For this review, take the finished solid that the model builds, in its own axes (mm). A direction names the side the tool comes from. Give positions to 0.01 mm unless a question says otherwise; leave off trailing zeros. Write each loop counter-clockwise with the first axis right and the second up, starting at its lowest first coordinate (ties: lowest second). Pieces come first, ordered by that corner, then holes. Notation, with made-up numbers: M -35.5,-2 L 23.5,-2 A14 cw 23.5,7 Z; hole C 5,41 d6. An arc over 180 degrees is marked long. Write item = value, one per line.
Autodesk Inventor part; units mm, degrees
ref_plane "YZ Plane" through (0, 0, 0) normal (1, 0, 0) x (0, 1, 0)
ref_plane "XZ Plane" through (0, 0, 0) normal (0, 1, 0) x (-1, 0, 0)
ref_plane "XY Plane" through (0, 0, 0) normal (0, 0, 1) x (1, 0, 0)
sketch "Boceto1" plane through (0, 0, 0) normal (0, 0, 1) x (1, 0, 0)
  line L0 (-32, -32) -> (32, -32)
  line L1 (32, -32) -> (32, 32)
  line L2 (32, 32) -> (-32, 32)
  line L3 (-32, 32) -> (-32, -32)
  line L4 (-32, -32) -> (32, 32) construction
  line L5 (32, -32) -> (-32, 32) construction
  point P0 (0, 0)
  dimension "d0" = 64
  dimension "d1" = 64
extrude "Extrusión1" add sketch "Boceto1" along normal blind 3
sketch "Boceto2" plane through (32, -32, 0) normal (1, 0, 0) x (0, 0, -1)
  line L0 (-74, 16.5) -> (1, 16.5)
  arc A0 (1, 10.5) -> (1, 16.5) centre (1, 13.5) ccw
  line L1 (1, 10.5) -> (-74, 10.5)
  line L2 (-74, -4.5) -> (-74, 10.5)
  line L3 (7, -4.5) -> (-74, -4.5)
  line L4 (7, -4.5) -> (7, 68.5)
  line L5 (7, 68.5) -> (-74, 68.5)
  line L6 (-74, 53.5) -> (-74, 68.5)
  line L7 (-74, 53.5) -> (1, 53.5)
  arc A1 (1, 47.5) -> (1, 53.5) centre (1, 50.5) ccw
  line L8 (1, 47.5) -> (-74, 47.5)
  line L9 (-74, 16.5) -> (-74, 47.5)
  line L10 (0, 0) -> (0, 64)
  line L11 (0, 64) -> (-3, 64)
  line L12 (-3, 0) -> (-3, 64)
  line L13 (0, 0) -> (-3, 0)
  line L14 (0, 47.5) -> (-3, 47.5)
  line L15 (-3, 47.5) -> (-3, 53.5)
  line L16 (-3, 53.5) -> (0, 53.5)
  line L17 (0, 53.5) -> (0, 47.5)
  line L18 (0, 47.7) -> (-3, 47.7)
  line L19 (-2.8, 47.7) -> (-2.8, 53.3)
  line L20 (-3, 53.3) -> (0, 53.3)
  line L21 (-0.2, 53.3) -> (-0.2, 47.7)
  line L22 (-2.5, 53) -> (-2.5, 48)
  line L23 (-3, 48) -> (0, 48)
  line L24 (-0.5, 48) -> (-0.5, 53)
  line L25 (0, 53) -> (-3, 53)
  point P0 (0, 32)
  dimension "d4" = 0.2
  dimension "d10" = 0.5
extrude "Extrusión2" add sketch "Boceto2" along normal blind 10 contours L12 L25 L19 L23 | L23 L21 L25 L10 | L19 L25 L22 L23 | L23 L24 L25 L21 | L22 L25 L24 L23
sketch "Boceto3" plane through (42, -32, 0) normal (1, 0, 0) x (0, 0, -1)
  line L0 (-3, 53) -> (-3, 48)
  line L1 (0, 48) -> (0, 53)
  line L2 (0, 47.7) -> (-3, 53.3)
  circle A0 centre (-1.5, 50.5) radius 5
  line L3 (-3, 53.3) -> (-3, 55.2697)
  line L4 (-3, 47.7) -> (0, 47.7)
  line L5 (0, 47.7) -> (0, 53.3)
  line L6 (0, 53.3) -> (-3, 53.3)
  line L7 (-3, 53.3) -> (-3, 47.7)
  line L8 (-3, 47.7) -> (-3, 42)
  line L9 (-3, 48) -> (0, 48)
  line L10 (0, 53) -> (-3, 53)
  point P0 (0, 32)
  point P1 (-3, 45.7303)
  point P2 (-2.8393, 53)
  point P3 (-0.1607, 48)
  dimension "d7" = 10
extrude "Extrusión3" add sketch "Boceto3" along normal blind 3 contours L10 L2 L9 L0 | L7 L2 L10 | L9 L2 L4 L7 | L6 L5 L10 L2 | L3 A0 L8 L4 L5 L1 L6 | L10 L1 L9 L2 | L9 L5 L2
ref_plane "Plano de trabajo1" through (0, -32, 3) normal (1, 0, 0) x (0, 0, -1)
ref_plane "Plano de trabajo2" through (-32, 0, 0) normal (0, 1, 0) x (1, 0, 0)
mirror "Simetría1" about plane through (-32, 0, 0) normal (0, 1, 0) of "Extrusión2", "Extrusión3"
mirror "Simetría2" about plane through (0, -32, 3) normal (1, 0, 0) of "Extrusión2", "Simetría1", "Extrusión3"
sketch "Boceto4" plane through (0, 0, 3) normal (0, 0, 1) x (1, 0, 0)
  arc A0 (-26.7524, -33.5) -> (-33.5, -26.7524) centre (-31.4, -31.4) ccw
  arc A1 (33.5, -26.7524) -> (26.7524, -33.5) centre (31.4, -31.4) ccw
  arc A2 (26.7524, 33.5) -> (33.5, 26.7524) centre (31.4, 31.4) ccw
  arc A3 (-33.5, 26.7524) -> (-26.7524, 33.5) centre (-31.4, 31.4) ccw
  line L0 (32, -32) -> (32, -21)
  line L1 (32, -21) -> (42, -21)
  line L2 (42, -23.2697) -> (42, -21)
  line L3 (42, -23.2697) -> (45, -23.2697)
  line L4 (45, -23.2697) -> (45, -13.7303)
  line L5 (42, -13.7303) -> (45, -13.7303)
  line L6 (42, -16) -> (42, -13.7303)
  line L7 (32, -16) -> (42, -16)
  line L8 (32, -16) -> (32, 16)
  line L9 (32, 16) -> (42, 16)
  line L10 (42, 16) -> (42, 13.7303)
  line L11 (42, 13.7303) -> (45, 13.7303)
  line L12 (45, 23.2697) -> (45, 13.7303)
  line L13 (42, 23.2697) -> (45, 23.2697)
  line L14 (42, 23.2697) -> (42, 21)
  line L15 (32, 21) -> (42, 21)
  line L16 (32, 21) -> (32, 32)
  line L17 (32, 32) -> (-32, 32)
  line L18 (-32, 32) -> (-32, 21)
  line L19 (-32, 21) -> (-42, 21)
  line L20 (-42, 23.2697) -> (-42, 21)
  line L21 (-42, 23.2697) -> (-45, 23.2697)
  line L22 (-45, 23.2697) -> (-45, 13.7303)
  line L23 (-42, 13.7303) -> (-45, 13.7303)
  line L24 (-42, 16) -> (-42, 13.7303)
  line L25 (-32, 16) -> (-42, 16)
  line L26 (-32, 16) -> (-32, -16)
  line L27 (-32, -16) -> (-42, -16)
  line L28 (-42, -16) -> (-42, -13.7303)
  line L29 (-42, -13.7303) -> (-45, -13.7303)
  line L30 (-45, -23.2697) -> (-45, -13.7303)
  line L31 (-42, -23.2697) -> (-45, -23.2697)
  line L32 (-42, -23.2697) -> (-42, -21)
  line L33 (-32, -21) -> (-42, -21)
  line L34 (-32, -21) -> (-32, -32)
  line L35 (-32, -32) -> (32, -32)
  arc A4 (-24.9298, -34.3235) -> (-34.3235, -24.9298) centre (-31.4, -31.4) ccw
  arc A5 (-34.3235, 24.9298) -> (-24.9298, 34.3235) centre (-31.4, 31.4) ccw
  arc A6 (24.9298, 34.3235) -> (34.3235, 24.9298) centre (31.4, 31.4) ccw
  arc A7 (34.3235, -24.9298) -> (24.9298, -34.3235) centre (31.4, -31.4) ccw
  point P0 (0, 0)
  point P1 (-32, 24.3254)
  point P2 (-24.3254, 32)
  point P3 (-24.3254, -32)
  point P4 (-32, -24.3254)
  point P5 (32, -24.3254)
  point P6 (24.3254, -32)
  point P7 (24.3254, 32)
  point P8 (32, 24.3254)
  dimension "d11" = 2
  dimension "d12" = 2
  dimension "d13" = 2
  dimension "d14" = 2
extrude "Extrusión4" cut sketch "Boceto4" against normal blind 3 contours L35 L34 A0 | A0 L34 A4 L35 | A7 L0 A1 L35 | A1 L0 L35 | L18 A3 L17 A5 | L18 L17 A3 | A6 L17 A2 L16 | A2 L17 L16
properties part number "Parte deslizante"
1. Machinability: for faces 1 (the face through (43.5, 18.6, -3.5)), 2 (the face through (-37, -16, 2)), 3 (the face through (-42, -18.6, -0.2)), 4 (the face through (37, -21, 2)), which of the approach directions +Z, -Z, +X, -X, +Y, -Y give a long, thin tool a straight path to every point of the face, cutting with its end or side? Answer none if there is none.
Responses:
face_1 = +X
face_2 = +Z, -Z
face_3 = -Z
face_4 = +Z, -Z, -Y
2. We need section A-A, the plane y = -18.5. Write out the cut boundary in (x, z).
Responses:
outline = M -45,-3.5 L -42,-3.5 L -42,0 L 42,0 L 42,-3.5 L 45,-3.5 L 45,3 L -45,3 Z
3. The part is to be moulded in two halves that separate along X. For faces 5 (the face through (0, -32, 1)), 6 (the face through (37, 16, 2)), say which applies: +X half, -X half, draft (parallel to the pull), parting line (faces both ways), or undercut.
Responses:
face_5 = draft
face_6 = undercut
4. For line 1 along X through (y, z) = (-14, 1); line 2 along X through (y, z) = (23, -0.25); line 3 along Y through (x, z) = (-36, 0.75), list the stretches that pass through material, from the lowest coordinate up. Write a range as from..to.
Responses:
line_1 = -45..-42, -32..32, 42..45
line_2 = -45..-42, 42..45
line_3 = -21..-16, 16..21
5. Insertion check: P1, Ø0.9, axis at x = -37.5, z = 1.5, coming from the -Y side; P2, Ø3.5, axis at x = 35.5, z = 2, coming from the +Y side; P3, Ø1.5, axis at y = 11, z = 0.5, coming from the -X side. Each pin has a flat end and moves straight along its axis. Give the tip position at first contact, or say it passes through.
Responses:
P1 = -21
P2 = 21
P3 = -32
6. We need section B-B, the plane x = -18. Write out the cut boundary in (y, z).
Responses:
outline = M -32,0 L 32,0 L 32,3 L -32,3 Z
